Can you work these out from the model? Positions are in its coordinate system, mm. Face numbers are marked on the shaded views. A direction names the side the tool comes from. Round coordinates to 2 decimals unless told otherwise and drop trailing zeros. Loops run counter-clockwise (first coordinate to the right, second up) from the corner with the lowest first, then second, coordinate; pieces in that order, holes last.
(1) If I drill on line 1 along Y through (x, z) = (0, 7); line 2 along X through (y, z) = (27, 64.5); line 3 along Z through (x, y) = (0.5, 27.5), over which ranges is the centre line in solid material (lowest first)?
(2) I want a section at C-C on y = -8.5. Write out the boundary of the cut face in (x, z).
(3) Will these pins go through, and if not, where does the flat tip stop? pin 1 Ø4 at (y, z) = (36.5, 63.5) entering from -X; pin 2 Ø5 at (x, z) = (-2.5, 60) entering from +Y; pin 3 Ø7 at (x, y) = (0, -8.5) entering from -Z.
(4) I want a section at B-B on x = 0. Write out the boundary of the cut face in (y, z).
(5) Which directions (+Z, -Z, +X, -X, +Y, -Y) give clear straight access to the entire face, cutting with the end or side of a thin tool? Please do the marked faces 5 and 6.
(6) Thinking about a two-plate mould opening in X: for the marked faces 1, 2, 3 and 4, which applies, released by +X, released by -X, zero draft, split by the parting line, or undercut?
(7) I want a section at A-A on z = 25. Write out the boundary of the cut face in (x, y) (3 decimals).
from build123d import *

# Parameters (mm, degrees)
F0_R     = 4.5
F1_DEPTH = 102.5
F2_DEPTH = 3.5
F3_DEPTH = 30
F4_DEPTH = 102.5
F6_DEPTH = 10
F7_R     = 6


with BuildPart() as f1:
    # F0 (on Top) → F1 (new body)
    with BuildSketch(Plane.XY):
        with BuildLine():
            ThreePointArc((21.343557, 34.00853), (0, 37.204707), (-21.343557, 34.00853))
            ThreePointArc((-21.343557, 34.00853), (-20.883556, 15.456117), (-14.112868, -1.822812))
            Line((-14.112868, -1.822812), (-7.232334, -12.965798))
            ThreePointArc((-7.232334, -12.965798), (-0.040256, -16.999905), (7.18971, -13.034101))
            Line((7.18971, -13.034101), (14.112868, -1.822812))
            ThreePointArc((14.112868, -1.822812), (20.883556, 15.456117), (21.343557, 34.00853))
        make_face()
        with Locations((0, -8.5)):
            Circle(F0_R, mode=Mode.SUBTRACT)
        with BuildLine():
            Line((11.125, 0), (0, 0))
            Line((0, 0), (-11.125, 0))
            ThreePointArc((-11.125, 0), (-17.220948, 15.062302), (-18.164667, 31.283983))
            ThreePointArc((-18.164667, 31.283983), (0, 33.704707), (18.164667, 31.283983))
            ThreePointArc((18.164667, 31.283983), (17.220948, 15.062302), (11.125, 0))
        make_face(mode=Mode.SUBTRACT)
        with Locations((0, -8.5)):
            Circle(F0_R)
    extrude(amount=F1_DEPTH)

    # F0 (on Top) → F2 (join)
    with BuildSketch(Plane.XY):
        with BuildLine():
            Line((-11.125, 0), (0, 0))
            Line((0, 0), (11.125, 0))
            ThreePointArc((11.125, 0), (17.220948, 15.062302), (18.164667, 31.283983))
            ThreePointArc((18.164667, 31.283983), (0, 33.704707), (-18.164667, 31.283983))
            ThreePointArc((-18.164667, 31.283983), (-17.220948, 15.062302), (-11.125, 0))
        make_face()
    extrude(amount=F2_DEPTH)

    # F0 (on Top) → F3 (cut)
    with BuildSketch(Plane.XY):
        with Locations((0, -8.5)):
            Circle(F0_R)
    extrude(amount=F3_DEPTH, mode=Mode.SUBTRACT)

    # F0 (on Top) → F4 (join)
    with BuildSketch(Plane.XY):
        with BuildLine():
            Line((-21.343557, 39.146077), (-21.343557, 34.00853))
            ThreePointArc((-21.343557, 34.00853), (0, 37.204707), (21.343557, 34.00853))
            Line((21.343557, 34.00853), (21.343557, 39.146077))
            Line((21.343557, 39.146077), (-21.343557, 39.146077))
        make_face()
    extrude(amount=F4_DEPTH)

    # F5 (on face) → F6 (cut)
    with BuildSketch(Plane(origin=(0, 39.146077, 0), x_dir=(-1, 0, 0), z_dir=(0, 1, 0))):
        Polygon((0, 89), (-17.75, 71.25), (0, 53.5), (17.75, 71.25), align=None)
    extrude(amount=-F6_DEPTH, mode=Mode.SUBTRACT)

    # F7
    f7_edges = [f1.edges().sort_by_distance(p)[0] for p in [
        (-17.75, 35.270601, 71.25),
        (0, 36.425392, 53.5),
        (17.75, 35.270601, 71.25),
        (0, 36.425392, 89),
    ]]
    fillet(f7_edges, radius=F7_R)


solid = f1.part
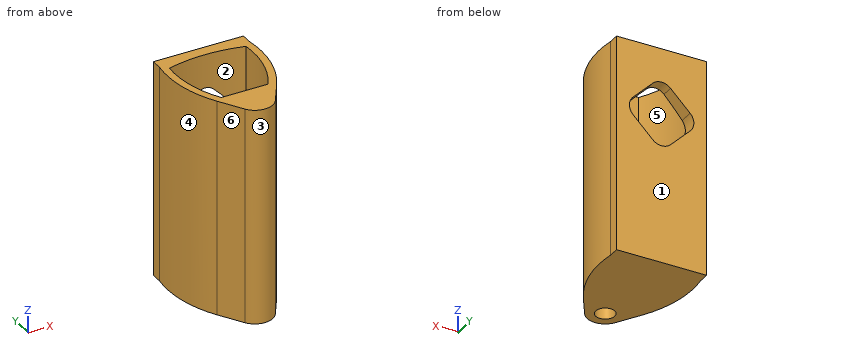
Filled sheet:
1. line 1: y = -17 to -13, -4 to 0, 33.7 to 39.15
1. line 2: x = -21.93 to -18.43, 18.43 to 21.93
1. line 3: z = 0 to 3.5
2. outline: (-9.99, 0) - (-4.5, 0) - (-4.5, 30) - (4.5, 30) - (4.5, 0) - (9.99, 0) - (9.99, 102.5) - (-9.99, 102.5) - close
3. pin 1: stops at x = -21.34
3. pin 2: stops at y = 0
3. pin 3: stops at z = 30
4. outline: (-17, 0) - (-13, 0) - (-13, 30) - (-4, 30) - (-4, 0) - (39.15, 0) - (39.15, 55.99) - (33.7, 55.99) - (33.7, 3.5) - (0, 3.5) - (0, 102.5) - (-17, 102.5) - close; (33.7, 86.51) - (39.15, 86.51) - (39.15, 102.5) - (33.7, 102.5) - close
5. face 5: +Z
5. face 6: +Z, -Z, -X, -Y
6. face 1: zero draft
6. face 2: undercut
6. face 3: split by the parting line
6. face 4: released by -X
7. outline: (-21.344, 34.009) arc R53.496 ccw to (-14.113, -1.823) - (-7.232, -12.966) arc R8.5 ccw to (7.19, -13.034) - (14.113, -1.823) arc R53.496 ccw to (21.344, 34.009) - (21.344, 39.146) - (-21.344, 39.146) - close; hole (-18.165, 31.284) arc R49.996 ccw to (-11.125, 0) - (11.125, 0) arc R49.996 ccw to (18.165, 31.284) arc R69.363 ccw to start; hole circle Ø9 at (0, -8.5)
